Can you work these out from the model? Positions are in its coordinate system, mm. A direction names the side the tool comes from. Round coordinates to 2 decimals unless told otherwise and drop trailing zeros. Order: outer loops, then holes, each group sorted by start corner. A loop starts at its lowest first (then second) coordinate and runs counter-clockwise, first axis right, second up. Notation, with made-up numbers: (-20.5, 34.25) -> (15.5, 34.25) arc R22 ccw to (15.5, 60.25) -> close; hole circle Ø9 at (30, 79.5). An arc over 180 degrees is marked (long way). Use a Markdown table: item, result. Add a question column.
Q1. For faces 5 (the face through (-49.37, -4.93, 43.68)), 6 (the face through (-61, -10, 1)), 7 (the face through (15, 8, -12)), which set-ups out of +Z, -Z, +X, -X, +Y, -Y let a thin tool reach every point of the face, with its end or its side?
Q2. If we section it at D-D on x = 71: List the corners of the cut face in (y, z) for me.
Q3. We'd pull the mould along Z, two halves only. Please class faces 1 (the face through (-7.21, 4.76, -32.45)), 2 (the face through (23, -15, 25)), 3 (the face through (-85, -5, -65)), 4 (the face through (47.539, -4.93, 44.346)): +Z half, -Z half, draft (parallel to the pull), parting line (faces both ways), or undercut.
Q4. If we section it at B-B on y = 3: List the corners of the cut face in (x, z) for me.
Q5. I need wall thicknesses on line 1 along Z through (x, y) = (0, -13); line 2 along Z through (x, y) = (0, -1); line 3 along Z through (x, y) = (0, 10.35). Which ranges of each line are inside material? Lowest first, please. Write a range as [from, to].
Q6. I'm going to push flat-ended pins straight in: pin 1 Ø9 at (x, z) = (51, -51) entering from -Y; pin 2 Ø1.5 at (x, y) = (28.5, 4) entering from +Z; pin 3 Ø10 at (x, z) = (-69.5, -28.5) entering from +Y; pin 4 Ø12 at (y, z) = (4.5, 15.5) entering from +X. Where does each tip first touch, or does it pass through?
Q7. If we section it at A-A on x = 0: Give the number of separate pieces and of enclosed holes in the cut face, plus the area to 3 significant figures.
```python
from build123d import *

# Parameters (mm, degrees)
F0_W          = 180
F0_H          = 140
F0_R          = 55
F1_DEPTH      = 10
F0_R_2        = 33
F2_DEPTH      = 15
F0_R_3        = 19
F3_DEPTH      = 25
F3_DEPTH_BACK = 15
F4_R          = 21
F4_R_2        = 19
F5_DEPTH      = 30
F6_R          = 22.5
F6_R_2        = 19
F7_DEPTH      = 7
F9_D          = 15
F11_D         = 5
F12_SIZE2     = 10
F12_SIZE      = 10
F13_SIZE2     = 5
F13_SIZE      = 5
F14_SIZE2     = 2
F14_SIZE      = 2
F15_SIZE2     = 1
F15_SIZE      = 1


with BuildPart() as f1:
    # F0 (on Front) → F1 (new body)
    with BuildSketch(Plane.XZ):
        Rectangle(F0_W, F0_H)
        Circle(F0_R, mode=Mode.SUBTRACT)
    extrude(amount=F1_DEPTH)

    # F0 (on Front) → F2 (join)
    with BuildSketch(Plane.XZ):
        Circle(F0_R)
        Circle(F0_R_2, mode=Mode.SUBTRACT)
    extrude(amount=F2_DEPTH)

    # F0 (on Front) → F3 (join, two sides)
    with BuildSketch(Plane.XZ) as f3_sk:
        Circle(F0_R_2)
        Circle(F0_R_3, mode=Mode.SUBTRACT)
    extrude(amount=F3_DEPTH)
    extrude(f3_sk.sketch, amount=-F3_DEPTH_BACK)

    # F4 (on face) → F5 (cut)
    with BuildSketch(Plane.XZ.offset(25)):
        Circle(F4_R)
        Circle(F4_R_2, mode=Mode.SUBTRACT)
    extrude(amount=-F5_DEPTH, mode=Mode.SUBTRACT)

    # F6 (on face) → F7 (cut)
    with BuildSketch(Plane(origin=(0, 15, 0), x_dir=(-1, 0, 0), z_dir=(0, 1, 0))):
        Circle(F6_R)
        Circle(F6_R_2, mode=Mode.SUBTRACT)
    extrude(amount=-F7_DEPTH, mode=Mode.SUBTRACT)

    # F9 (through all)
    with Locations(Plane.XZ.offset(10)):
        with Locations((-51, 51), (51, 51), (51, -51), (-51, -51)):
            Hole(F9_D / 2)

    # F11 (through all)
    with Locations(Plane.XZ.offset(15)):
        with Locations((0, -42)):
            Hole(F11_D / 2)

    # F12
    f12_edges = [f1.edges().sort_by_distance(p)[0] for p in [
        (-90, -5, 70),
        (-90, -5, -70),
        (90, -5, 70),
        (90, -5, -70),
    ]]
    chamfer(f12_edges, length=F12_SIZE, length2=F12_SIZE2)

    # F13
    f13_edges = [f1.edges().sort_by_distance(p)[0] for p in [
        (-33, 0, 0),
    ]]
    chamfer(f13_edges, length=F13_SIZE, length2=F13_SIZE2)

    # F14
    f14_edges = [f1.edges().sort_by_distance(p)[0] for p in [
        (-33, 15, 0),
    ]]
    chamfer(f14_edges, length=F14_SIZE, length2=F14_SIZE2)

    # F15
    f15_edges = [f1.edges().sort_by_distance(p)[0] for p in [
        (22.5, 15, 0),
        (-21, -25, 0),
        (-33, -25, 0),
        (-55, -15, 0),
    ]]
    chamfer(f15_edges, length=F15_SIZE, length2=F15_SIZE2)


solid = f1.part
```
Answer below:
| question | item | result |
|---|---|---|
| 1 | face 5 | +Y, -Y |
| 1 | face 6 | -Y |
| 1 | face 7 | +Y |
| 2 | outline | (-10, -70) -> (0, -70) -> (0, 70) -> (-10, 70) -> close |
| 3 | face 1 | parting line |
| 3 | face 2 | draft |
| 3 | face 3 | -Z half |
| 3 | face 4 | undercut |
| 4 | outline | circle Ø70 at (0, 0); hole circle Ø42 at (0, 0) |
| 5 | line 1 | [-55, -44.5], [-39.5, -21], [21, 55] |
| 5 | line 2 | [-70, -44.5], [-39.5, -21], [21, 70] |
| 5 | line 3 | [-33, -22.5], [22.5, 33] |
| 6 | pin 1 | through |
| 6 | pin 2 | z = 20.26 |
| 6 | pin 3 | y = 0 |
| 6 | pin 4 | x = 90 |
| 7 | separate pieces | 3 |
| 7 | enclosed holes | 0 |
| 7 | area | 1,850 mm² |
